```python
from build123d import *

# Parameters (mm, degrees)
F0_W   = 2.54
F0_H   = 6.35
F0_H_2 = 2.54
F0_W_2 = 39.37
F0_W_3 = 6.35
F0_H_3 = 2.5146
F0_H_4 = 1.2446


# Not quite as in the source:
# - a feature names something its author has since deleted; it is built from what else it names


with BuildPart() as f1:
    # F0 (on Front) → F1 (revolve)
    with BuildSketch(Plane.XZ):
        Polygon((44.45, 12.7), (41.91, 12.7), (41.91, 6.35), (44.45, 6.35), (44.45, 7.5946), (44.45, 10.1854), align=None)
        with Locations((40.64, 9.525)):
            Rectangle(F0_W, F0_H)
        with Locations((40.64, 13.97)):
            Rectangle(F0_W, F0_H_2)
        with Locations((19.685, 9.525)):
            Rectangle(F0_W_2, F0_H)
        with Locations((47.625, 11.4427)):
            Rectangle(F0_W_3, F0_H_3)
        with Locations((47.625, 6.9723)):
            Rectangle(F0_W_3, F0_H_4)
    revolve(axis=Axis((19.685, 0, 6.35), (1, 0, 0)))


solid = f1.part
```
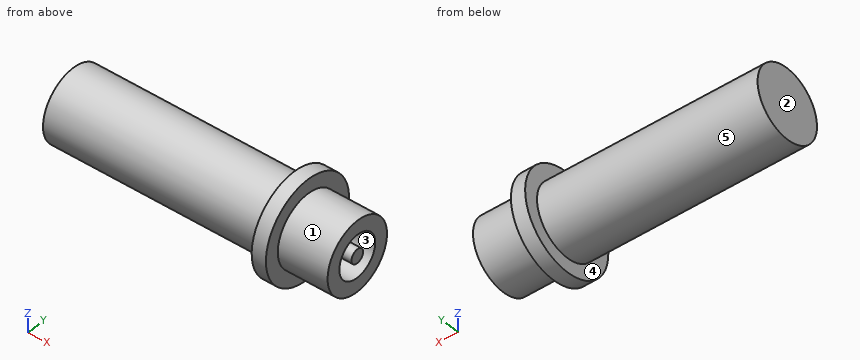
Could you check a few things on this model? Use its own coordinates, in mm. Face numbers are marked on the shaded views. A direction names the side the tool comes from. Round coordinates to 2 decimals unless told otherwise and drop trailing zeros. Loops run counter-clockwise (first coordinate to the right, second up) from the corner with the lowest first, then second, coordinate; pieces in that order, holes last. Notation, with made-up numbers: (46, 56.25) - (94, 56.25) arc R22 cw to (94, 84.25) - close; hole circle Ø7 at (30.5, 79.5). An arc over 180 degrees is marked (long way). Answer in a Markdown table with one row per item. Add a question column.
(1) If we section it at A-A (y = 0): Please give me the cut outline in (x, z), plus the area to 3 significant figures.
(2) For the marked faces 1 and 2, which set-ups out of +Z, -Z, +X, -X, +Y, -Y let a thin tool reach every point of the face, with its end or its side?
(3) I need wall thicknesses on line 1 along Z through (x, y) = (47, 0); line 2 along Y through (x, z) = (46.25, 6.35); line 3 along X through (y, z) = (8, 7.25). Which ranges of each line are inside material? Lowest first, please.
(4) If we section it at D-D (z = 8.75): Please give me the cut outline in (x, y).
(5) I'm going to push flat-ended pins straight in: pin 1 (6 mm diameter, centred on x = 27, y = -6.5, fed in from +Z); pin 2 (1.5 mm diameter, centred on x = 17.5, y = 5, fed in from +Z); pin 3 (3 mm diameter, centred on x = 25.5, y = 2.5, fed in from +Z). Where does each tip first touch, or does it pass through?
(6) If we section it at C-C (x = 37.5): Please give me the cut outline in (y, z).
(7) If we mould it in two halves opening along Z, with no side actions, what happens to the marked faces 3, 4 and 5? For each: pulls with the +Z half, pulls with the -Z half, needs draft (parallel to the pull), parting line crosses it, or undercut.
(8) If we section it at B-B (z = 6.35): Please give me the cut outline in (x, y).
Model answer:
| question | item | result |
|---|---|---|
| 1 | outline | (0, 0) - (39.37, 0) - (39.37, -2.54) - (41.91, -2.54) - (41.91, 0) - (50.8, 0) - (50.8, 2.51) - (44.45, 2.51) - (44.45, 5.11) - (50.8, 5.11) - (50.8, 7.59) - (44.45, 7.59) - (44.45, 10.19) - (50.8, 10.19) - (50.8, 12.7) - (41.91, 12.7) - (41.91, 15.24) - (39.37, 15.24) - (39.37, 12.7) - (0, 12.7) - close |
| 1 | area | 625 mm² |
| 2 | face 1 | +X |
| 2 | face 2 | +Z, -Z, -X, +Y, -Y |
| 3 | line 1 | z = 0 to 2.51, 5.11 to 7.59, 10.19 to 12.7 |
| 3 | line 2 | y = -6.35 to -3.84, -1.24 to 1.24, 3.84 to 6.35 |
| 3 | line 3 | x = 39.37 to 41.91 |
| 4 | outline | (0, -5.88) - (39.37, -5.88) - (39.37, -8.56) - (41.91, -8.56) - (41.91, -5.88) - (50.8, -5.88) - (50.8, -2.99) - (44.45, -2.99) - (44.45, 2.99) - (50.8, 2.99) - (50.8, 5.88) - (41.91, 5.88) - (41.91, 8.56) - (39.37, 8.56) - (39.37, 5.88) - (0, 5.88) - close |
| 5 | pin 1 | stops at z = 11.65 |
| 5 | pin 2 | stops at z = 11.07 |
| 5 | pin 3 | stops at z = 12.62 |
| 6 | outline | circle Ø12.7 at (0, 6.35) |
| 7 | face 3 | undercut |
| 7 | face 4 | needs draft |
| 7 | face 5 | parting line crosses it |
| 8 | outline | (0, -6.35) - (39.37, -6.35) - (39.37, -8.89) - (41.91, -8.89) - (41.91, -6.35) - (50.8, -6.35) - (50.8, -3.84) - (44.45, -3.84) - (44.45, -1.24) - (50.8, -1.24) - (50.8, 1.24) - (44.45, 1.24) - (44.45, 3.84) - (50.8, 3.84) - (50.8, 6.35) - (41.91, 6.35) - (41.91, 8.89) - (39.37, 8.89) - (39.37, 6.35) - (0, 6.35) - close |
